CAD build for the part. Positions are in the model's coordinates, mm. A direction names the side the tool comes from. Round coordinates to 2 decimals unless told otherwise and drop trailing zeros. Loops run counter-clockwise (first coordinate to the right, second up) from the corner with the lowest first, then second, coordinate; pieces in that order, holes last.
```python
from build123d import *

# Parameters (mm, degrees)
F0_R     = 1.5930121089
F0_R_2   = 1.27
F1_DEPTH = 12.7
F0_W     = 7.9617746973
F0_H     = 11.1195407808
F0_W_2   = 65.5765477568
F0_H_2   = 13.5095529258
F2_DEPTH = 25.4
F3_SIZE  = 7.62
F5_D     = 3.5814
F6_R     = 2.54


with BuildPart() as f1:
    # F0 (on Top) → F1 (new body)
    with BuildSketch(Plane.XY):
        Polygon((-11.4968402433, 18.5921955854), (-0.2459318388, 18.5921955854), (36.7631597567, 18.5921955854), (44.724934454, 18.5921955854), (44.8390953243, 18.5921955854), (44.8390953243, 41.7590104043), (-20.7374524325, 41.7590104043), (-20.7374524325, 18.5921955854), align=None)
        Polygon((-11.4968402433, 13.8334799558), (-11.4968402433, 18.5921955854), (-20.7374524325, 18.5921955854), (-20.7374524325, -18.1194674224), (-11.4968402433, -18.1194674224), align=None)
        with Locations((-16.2880346179, 13.6660579592)):
            Circle(F0_R, mode=Mode.SUBTRACT)
        Polygon((44.724934454, 18.5921955854), (36.7631597567, 18.5921955854), (36.7631597567, 13.8334799558), (36.7631597567, -18.1194674224), (44.724934454, -18.1194674224), align=None)
        with Locations((40.6009033322, 13.8249658048)):
            Circle(F0_R_2, mode=Mode.SUBTRACT)
        with Locations((40.6009033322, 13.8249658048)):
            Circle(F0_R_2)
        with Locations((-16.2880346179, 13.6660579592)):
            Circle(F0_R)
    extrude(amount=F1_DEPTH)

    # F0 (on Top) → F2 (join)
    with BuildSketch(Plane.XY):
        Polygon((-11.4968402433, -29.2390082031), (-11.4968402433, -18.1194674224), (-20.7374524325, -18.1194674224), (-20.7374524325, -29.0999621163), (-14.0633266419, -29.2390082031), align=None)
        with Locations((40.7440471053, -23.6792378128)):
            Rectangle(F0_W, F0_H)
        with Locations((12.0508214459, 48.5137868673)):
            Rectangle(F0_W_2, F0_H_2)
    extrude(amount=F2_DEPTH)

    # F3
    f3_edges = [f1.edges().sort_by_distance(p)[0] for p in [
        (-16.117146, -18.119467, 25.4),
        (40.744047, -18.119467, 25.4),
    ]]
    chamfer(f3_edges, length=F3_SIZE)

    # F5 (through all)
    with Locations(Plane.XZ):
        with Locations((30.9119317681, 16.3051951677), (-4.1159610264, 16.3051951677)):
            Hole(F5_D / 2)

    # F6
    f6_edges = [f1.edges().sort_by_distance(p)[0] for p in [
        (-11.49684, 0.236364, 12.7),
        (12.63316, 18.592196, 12.7),
        (36.76316, 0.236364, 12.7),
    ]]
    fillet(f6_edges, radius=F6_R)


solid = f1.part
```
Item 1: Probe line 1 (X direction, y = -18, z = 6); line 2 (Z direction, x = 41, y = -10.5); line 3 (Y direction, x = 11, z = 13). List the from-to ranges inside material, lowest first.
Answers follow:
line 1: x = -20.74 to -11.5, 36.76 to 44.72
line 2: z = 0 to 12.7
line 3: y = 41.76 to 55.27
Item 2: Cut at B-B, the plane y = 14.5. Give the cut face in (x, z), plus the area to 3 significant figures.
Answers follow:
outline: (-20.74, 0) - (-11.5, 0) - (-11.5, 10.16) arc R2.54 ccw to (-14.04, 12.7) - (-20.74, 12.7) - close; (36.76, 0) - (44.72, 0) - (44.72, 12.7) - (39.3, 12.7) arc R2.54 ccw to (36.76, 10.16) - close
area: 216 mm2
Item 3: Flat gauge pins, fed straight in: P1, Ø14, axis at x = 27, z = 18.5, coming from the -Y side; P2, Ø5, axis at x = 18.5, z = 4, coming from the -Y side; P3, Ø8, axis at y = 31, z = 18, coming from the +X side; P4, Ø4.5, axis at x = 30.91, z = 16.31, coming from the -Y side. Where does each tip first touch, or does it go through?
Answers follow:
P1: stops at y = 18.97
P2: stops at y = 18.59
P3: passes through
P4: stops at y = 41.76
Item 4: Two-plate mould, pull along Y, no slides. Class faces 1 (the flat face through (12, 41.759, 19)), 2 (the flat face through (12, 55.269, 13)), 3 (the flat face through (12, 49, 25.4)): released by +Y, released by -Y, zero draft, split by the parting line, or undercut.
Answers follow:
face 1: undercut
face 2: released by +Y
face 3: zero draft
Item 5: Cut at C-C, the plane x = 40.5. Give the cut face in (y, z), plus the area to 3 significant figures.
Answers follow:
outline: (-29.24, 0) - (55.27, 0) - (55.27, 25.4) - (41.76, 25.4) - (41.76, 12.7) - (-18.12, 12.7) - (-18.12, 17.78) - (-25.74, 25.4) - (-29.24, 25.4) - close
area: 1,360 mm2
Item 6: Cut at A-A, the plane z = 23. Give the cut face in (x, y), plus the area to 3 significant figures.
Answers follow:
outline: (-20.74, -29.1) - (-14.06, -29.24) - (-11.5, -29.24) - (-11.5, -23.34) - (-20.74, -23.34) - close; (-20.74, 41.76) - (44.84, 41.76) - (44.84, 55.27) - (-20.74, 55.27) - close; (36.76, -29.24) - (44.72, -29.24) - (44.72, -23.34) - (36.76, -23.34) - close
area: 987 mm2
Item 7: 3-axis set-ups, long thin cutter, end or side, ignore diameter. For faces 4 (the flat face through (-13, -29.239, 13)), 5 (the flat face through (-20.737, 14, 10)), 6 (the flat face through (36.763, -10, 7)), 7 (the flat face through (-16.05, -21.98, 21.64)), 8 (the cylindrical face through (37.53, 1.23, 11.98)): which of +Z, -Z, +X, -X, +Y, -Y reach the whole face in a straight line?
Answers follow:
face 4: +Z, -Z, +X, -X, -Y
face 5: +Z, -Z, -X, +Y, -Y
face 6: +Z, -Z, -Y
face 7: +Z, +X, -X
face 8: +Z
Item 8: Cut at D-D, the plane y = 31. Give the cut face in (x, z).
Answers follow:
outline: (-20.74, 0) - (44.84, 0) - (44.84, 12.7) - (-20.74, 12.7) - close
